Can you work these out from the model? Positions are in its coordinate system, mm. Face numbers are marked on the shaded views. Give positions to 0.01 mm unless a question says otherwise; leave off trailing zeros. Loops run counter-clockwise (first coordinate to the right, second up) from the corner with the lowest first, then second, coordinate; pieces in that order, holes last. Notation, with made-up numbers: (-23.75, 82.25) - (-16.75, 82.25) arc R18 cw to (-16.75, 98.25) - close; hole circle Ø1 at (-39, -35.5). An arc over 180 degrees is marked (long way). Answer in a Markdown table with one row per item.
from build123d import *

# Parameters (mm, degrees)
SKETCH_1_W          = 90
SKETCH_1_H          = 150
SKETCH_1_R          = 2
SKETCH_1_R_2        = 2.15
SKETCH_1_R_3        = 1.6
EXTRUDE_1_DEPTH     = 5
FILLET_1_R          = 8
SKETCH_2_R          = 3.6
CUT_EXTRUDE_1_DEPTH = 2
SKETCH_4_R          = 30
EXTRUDE_2_DEPTH     = 4


with BuildPart() as part:
    # 草图1 → 凸台-拉伸1 (new body)
    with BuildSketch(Plane.XY):
        with Locations((45, -75)):
            Rectangle(SKETCH_1_W, SKETCH_1_H)
        with Locations((79, -60)):
            Circle(SKETCH_1_R, mode=Mode.SUBTRACT)
        with Locations((79, -90)):
            Circle(SKETCH_1_R, mode=Mode.SUBTRACT)
        with Locations((49, -60)):
            Circle(SKETCH_1_R, mode=Mode.SUBTRACT)
        with Locations((49, -90)):
            Circle(SKETCH_1_R, mode=Mode.SUBTRACT)
        with Locations((40.5, -39.5)):
            Circle(SKETCH_1_R_2, mode=Mode.SUBTRACT)
        with Locations((40.5, -110.5)):
            Circle(SKETCH_1_R_2, mode=Mode.SUBTRACT)
        with Locations((76, -75)):
            Circle(SKETCH_1_R_2, mode=Mode.SUBTRACT)
        with Locations((5, -75)):
            Circle(SKETCH_1_R_2, mode=Mode.SUBTRACT)
        with Locations((85, -117.5)):
            Circle(SKETCH_1_R_3, mode=Mode.SUBTRACT)
        with Locations((75, -117.5)):
            Circle(SKETCH_1_R_3, mode=Mode.SUBTRACT)
        with Locations((65, -117.5)):
            Circle(SKETCH_1_R_3, mode=Mode.SUBTRACT)
        with Locations((55, -117.5)):
            Circle(SKETCH_1_R_3, mode=Mode.SUBTRACT)
        with Locations((45, -117.5)):
            Circle(SKETCH_1_R_3, mode=Mode.SUBTRACT)
        with Locations((85, -32.5)):
            Circle(SKETCH_1_R_3, mode=Mode.SUBTRACT)
        with Locations((75, -32.5)):
            Circle(SKETCH_1_R_3, mode=Mode.SUBTRACT)
        with Locations((65, -32.5)):
            Circle(SKETCH_1_R_3, mode=Mode.SUBTRACT)
        with Locations((55, -32.5)):
            Circle(SKETCH_1_R_3, mode=Mode.SUBTRACT)
        with Locations((45, -32.5)):
            Circle(SKETCH_1_R_3, mode=Mode.SUBTRACT)
        with Locations((35, -117.5)):
            Circle(SKETCH_1_R_3, mode=Mode.SUBTRACT)
        with Locations((25, -117.5)):
            Circle(SKETCH_1_R_3, mode=Mode.SUBTRACT)
        with Locations((15, -117.5)):
            Circle(SKETCH_1_R_3, mode=Mode.SUBTRACT)
        with Locations((35, -32.5)):
            Circle(SKETCH_1_R_3, mode=Mode.SUBTRACT)
        with Locations((25, -32.5)):
            Circle(SKETCH_1_R_3, mode=Mode.SUBTRACT)
        with Locations((15, -32.5)):
            Circle(SKETCH_1_R_3, mode=Mode.SUBTRACT)
        with Locations((8, -117.5)):
            Circle(SKETCH_1_R_3, mode=Mode.SUBTRACT)
        with Locations((8, -32.5)):
            Circle(SKETCH_1_R_3, mode=Mode.SUBTRACT)
        with Locations((36.5, -4)):
            Circle(SKETCH_1_R_3, mode=Mode.SUBTRACT)
        with Locations((36.5, -13)):
            Circle(SKETCH_1_R_3, mode=Mode.SUBTRACT)
        with Locations((36.5, -137)):
            Circle(SKETCH_1_R_3, mode=Mode.SUBTRACT)
        with Locations((36.5, -146)):
            Circle(SKETCH_1_R_3, mode=Mode.SUBTRACT)
        with Locations((55, -75)):
            Circle(SKETCH_1_R_3, mode=Mode.SUBTRACT)
        with Locations((40.5, -75)):
            Circle(SKETCH_1_R_3, mode=Mode.SUBTRACT)
    extrude(amount=EXTRUDE_1_DEPTH)

    # 圆角1
    fillet_1_edges = [part.edges().sort_by_distance(p)[0] for p in [
        (0, 0, 2.5),
        (90, 0, 2.5),
        (90, -150, 2.5),
        (0, -150, 2.5),
    ]]
    fillet(fillet_1_edges, radius=FILLET_1_R)

    # 草图2 → 切除-拉伸1 (cut)
    with BuildSketch(Plane.XY.offset(5)):
        with Locations((40.5, -39.5)):
            Circle(SKETCH_2_R)
        with Locations((76, -75)):
            Circle(SKETCH_2_R)
        with Locations((5, -75)):
            Circle(SKETCH_2_R)
        with Locations((40.5, -110.5)):
            Circle(SKETCH_2_R)
    extrude(amount=-CUT_EXTRUDE_1_DEPTH, mode=Mode.SUBTRACT)

    # 草图4 → 凸台-拉伸2 (add)
    with BuildSketch(Plane(origin=(0, 0, 0), x_dir=(-1, 0, 0), z_dir=(0, 0, -1))):
        with BuildLine():
            ThreePointArc((-42.199612772, -35.036124857), (-68.784271247, -46.715728753), (-80.463875143, -73.300387228))
            ThreePointArc((-80.463875143, -73.300387228), (-71.223509147, -75), (-80.463875143, -76.699612772))
            ThreePointArc((-80.463875143, -76.699612772), (-68.784271247, -103.284271247), (-42.199612772, -114.963875143))
            ThreePointArc((-42.199612772, -114.963875143), (-40.5, -105.723509147), (-38.800387228, -114.963875143))
            ThreePointArc((-38.800387228, -114.963875143), (-12.215728753, -103.284271247), (-0.536124857, -76.699612772))
            ThreePointArc((-0.536124857, -76.699612772), (-9.776490853, -75), (-0.536124857, -73.300387228))
            ThreePointArc((-0.536124857, -73.300387228), (-12.215728753, -46.715728753), (-38.800387228, -35.036124857))
            ThreePointArc((-38.800387228, -35.036124857), (-40.5, -44.276490853), (-42.199612772, -35.036124857))
        make_face()
        with Locations((-40.5, -75)):
            Circle(SKETCH_4_R, mode=Mode.SUBTRACT)
    extrude(amount=EXTRUDE_2_DEPTH)


solid = part.part
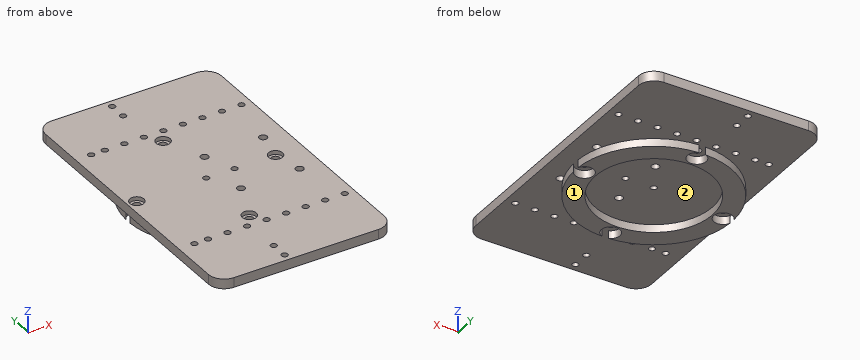
Q1. For pin 1 (5.5 mm diameter, centred on x = 5, y = -75, fed in from -Z), with a flat end and sliding along its axis, tell me the tip position at first contact or that it passes through.
Checked values:
| item | result |
|---|---|
| pin 1 | stops at z = 0 |
Q2. If I drill on line 1 (Y direction, x = 55, z = 2.75); line 2 (Y direction, x = 49, z = 3.35); line 3 (Z direction, x = 86, y = -13.5), over which ranges is the centre line in solid material (lowest first)? Write a range as [from, to].
Checked values:
| item | result |
|---|---|
| line 1 | y = [-150, -119.1], [-115.9, -76.6], [-73.4, -34.1], [-30.9, 0] |
| line 2 | y = [-150, -92], [-88, -62], [-58, 0] |
| line 3 | z = [0, 5] |
Q3. Imagine slicing it at B-B, the plane x = 20. Write out the boundary of the cut face in (y, z), and give its area (3 significant figures).
Checked values:
| item | result |
|---|---|
| outline | (-150, 0) - (-109.35, 0) - (-109.35, -4) - (-96.9, -4) - (-96.9, 0) - (-53.1, 0) - (-53.1, -4) - (-40.65, -4) - (-40.65, 0) - (0, 0) - (0, 5) - (-150, 5) - close |
| area | 850 mm² |
Q4. If we mould it in two halves opening along X, with no side actions, what happens to the marked faces 1 and 2? For each: released by +X, released by -X, zero draft, split by the parting line, or undercut.
Checked values:
| item | result |
|---|---|
| face 1 | zero draft |
| face 2 | undercut |
Q5. Imagine slicing it at C-C, the plane x = 30.5. Write out the boundary of the cut face in (y, z).
Checked values:
| item | result |
|---|---|
| outline | (-150, 0) - (-113.73, 0) - (-113.73, -4) - (-103.28, -4) - (-103.28, 0) - (-46.72, 0) - (-46.72, -4) - (-36.27, -4) - (-36.27, 0) - (0, 0) - (0, 5) - (-150, 5) - close |
Q6. Imagine slicing it at A-A, the plane y = -137. Write out the boundary of the cut face in (x, z).
Checked values:
| item | result |
|---|---|
| outline | (0, 0) - (34.9, 0) - (34.9, 5) - (0, 5) - close; (38.1, 0) - (90, 0) - (90, 5) - (38.1, 5) - close |
